Input: part model. Units: mm. Frame: model coordinates. Face numbers are marked on the shaded views. A direction names the side the tool comes from. Give positions to 0.01 mm unless a question says otherwise; leave off trailing zeros. Order: outer loops, then holes, each group sorted by start corner. A loop starts at its lowest first (then second) coordinate and runs counter-clockwise, first axis right, second up.
```python
from build123d import *

# Parameters (mm, degrees)
SKETCH1_W          = 36.5
SKETCH1_H          = 37.1
BODY_DEPTH         = 8
SKETCH2_W          = 2
SKETCH2_H          = 4
FEMALE_TABS_DEPTH  = 2
SKETCH3_W          = 1.8
SKETCH3_H          = 3.6
MALE_TABS_DEPTH    = 9
SKETCH5_W          = 17.9
SKETCH5_H          = 17.9
SIPM_WINDOW_DEPTH  = 8
SIPM_WINDOW_TAPER  = -10
CUT_EXTRUDE2_DEPTH = 6
SKETCH7_W          = 18.9
SKETCH7_H          = 2
RIGHT_DROP_DEPTH   = 3.24
SKETCH8_W          = 12.6
SKETCH8_H          = 2
LEFT_DROP_DEPTH    = 5.44


with BuildPart() as part:
    # Sketch1 → Body (new body)
    with BuildSketch(Plane(origin=(0, 0, 0), x_dir=(1, 0, 0), z_dir=(0, 1, 0))):
        with Locations((18.25, -18.55)):
            Rectangle(SKETCH1_W, SKETCH1_H)
    extrude(amount=BODY_DEPTH)

    # Sketch2 → Female Tabs (cut)
    with BuildSketch(Plane(origin=(0, 0, 0), x_dir=(-1, 0, 0), z_dir=(0, -1, 0))):
        with Locations((-1, -4.1)):
            Rectangle(SKETCH2_W, SKETCH2_H)
        with Locations((-35.5, -27.1)):
            Rectangle(SKETCH2_W, SKETCH2_H)
    extrude(amount=-FEMALE_TABS_DEPTH, mode=Mode.SUBTRACT)

    # Sketch3 → Male Tabs (add)
    with BuildSketch(Plane(origin=(0, 0, 0), x_dir=(-1, 0, 0), z_dir=(0, -1, 0))):
        with Locations((-0.9, -27.3)):
            Rectangle(SKETCH3_W, SKETCH3_H)
        with Locations((-35.6, -3.9)):
            Rectangle(SKETCH3_W, SKETCH3_H)
    extrude(amount=MALE_TABS_DEPTH)

    # Sketch5 → SiPM Window (cut)
    with BuildSketch(Plane(origin=(0, 0, 0), x_dir=(-1, 0, 0), z_dir=(0, -1, 0))):
        with Locations((-18.25, -11.45)):
            Rectangle(SKETCH5_W, SKETCH5_H)
    extrude(amount=-SIPM_WINDOW_DEPTH, taper=SIPM_WINDOW_TAPER, mode=Mode.SUBTRACT)

    # Sketch6 → Cut-Extrude2 (cut)
    with BuildSketch(Plane.XZ):
        Polygon((34, 1.5), (29.2, 1.5), (29.2, 22.4), (7.3, 22.4), (7.3, 1.5), (2.5, 1.5), (2.5, 35.1), (34, 35.1), align=None)
    extrude(amount=-CUT_EXTRUDE2_DEPTH, mode=Mode.SUBTRACT)

    # Sketch7 → Right Drop (add)
    with BuildSketch(Plane.XZ):
        with Locations((24.55, 36.1)):
            Rectangle(SKETCH7_W, SKETCH7_H)
    extrude(amount=RIGHT_DROP_DEPTH)

    # Sketch8 → Left Drop (add)
    with BuildSketch(Plane.XZ):
        with Locations((8.8, 36.1)):
            Rectangle(SKETCH8_W, SKETCH8_H)
    extrude(amount=LEFT_DROP_DEPTH)


solid = part.part
```
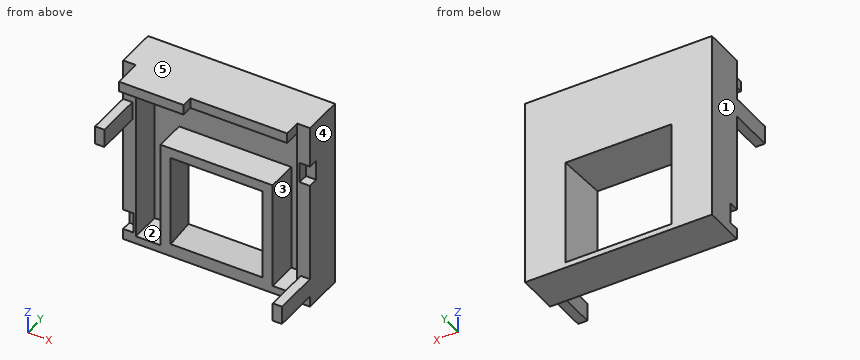
1) First-contact query: P1, Ø1.6, axis at x = 22, z = 35.5, coming from the -Y side; P2, Ø11, axis at x = 25.5, z = 18.5, coming from the -Y side; P3, Ø2, axis at x = 11.5, y = -7, coming from the +Z side; P4, Ø0.6, axis at y = -2.5, z = 35.5, coming from the -X side. Flat tips, straight axial feed; report the tip coordinate or a pass-through.
2) Cut plane B-B (y = -2.25). Return the cut outline in (x, z).
3) Cut plane C-C (y = 2.75). Count the separate pieces of the cut face and the enclosed holes in it, then the cut area to 3 significant figures.
4) Reachability of the marked faces 1 and 2 from +Z, -Z, +X, -X, +Y, -Y: full face, straight path, thin tool, end or side. Return the list, or none.
5) Line query: probe 1 along X at (y, z) = (3.5, 14.5); probe 2 along Z at (x, y) = (20.5, 1); probe 3 along X at (y, z) = (3.25, 33.5). Output: solid intervals per line, ascending.
6) Cut plane A-A (y = -7.25). Return the cut outline in (x, z).
7) Pull-direction query (X, two-part tool) for the marked faces 3, 4 and 5; classes: pulls with the +X half, pulls with the -X half, needs draft (parallel to the pull), parting line crosses it, or undercut.
Geometry says:
1. P1: stops at y = -3.24
1. P2: stops at y = 0
1. P3: passes through
1. P4: stops at x = 2.5
2. outline: (0, 25.5) - (1.8, 25.5) - (1.8, 29.1) - (0, 29.1) - close; (2.5, 35.1) - (34, 35.1) - (34, 37.1) - (2.5, 37.1) - close; (34.7, 2.1) - (36.5, 2.1) - (36.5, 5.7) - (34.7, 5.7) - close
3. separate pieces: 1
3. enclosed holes: 2
3. area: 397 mm2
4. face 1: +Z, -Z, -X, +Y, -Y
4. face 2: -Y
5. probe 1: x = 0 to 2.5, 7.3 to 8.68, 27.82 to 29.2, 34 to 36.5
5. probe 2: z = 0 to 2.32, 20.58 to 22.4, 35.1 to 37.1
5. probe 3: x = 0 to 2.5, 34 to 36.5
6. outline: (0, 25.5) - (1.8, 25.5) - (1.8, 29.1) - (0, 29.1) - close; (34.7, 2.1) - (36.5, 2.1) - (36.5, 5.7) - (34.7, 5.7) - close
7. face 3: undercut
7. face 4: pulls with the +X half
7. face 5: needs draft
